from build123d import *

# Parameters (mm, degrees)
F0_W     = 127
F0_H     = 63.5
F1_DEPTH = 12.7
F2_W     = 127
F2_H     = 12.7
F3_DEPTH = 44.45
F5_DEPTH = 57.15
F6_R     = 12.7
F7_DEPTH = 44.45
F8_R     = 5.08
F9_DEPTH = 25.4


with BuildPart() as f1:
    # F0 (on Front) → F1 (new body)
    with BuildSketch(Plane.XZ):
        with Locations((63.5, 31.75)):
            Rectangle(F0_W, F0_H)
    extrude(amount=F1_DEPTH)

    # F2 (on face) → F3 (join)
    with BuildSketch(Plane.XZ.offset(12.7)):
        with Locations((63.5, 6.35)):
            Rectangle(F2_W, F2_H)
    extrude(amount=F3_DEPTH)

    # F4 (on face) → F5 (join)
    with BuildSketch(Plane.XZ.offset(57.15)):
        Polygon((31.75, -21.59), (63.5, -21.59), (95.25, -21.59), (95.25, -11.3792), (76.2, -11.3792), (76.2, 0), (63.5, 0), (50.8, 0), (50.8, -11.3792), (31.75, -11.3792), align=None)
    extrude(amount=-F5_DEPTH)

    # F6 (on face) → F7 (join)
    with BuildSketch(Plane.XZ.offset(57.15)):
        with BuildLine():
            Line((42.406574, 52.250173), (15.875, 12.7))
            Line((15.875, 12.7), (111.125, 12.7))
            Line((111.125, 12.7), (84.593426, 52.250173))
            ThreePointArc((84.593426, 52.250173), (63.5, 63.5), (42.406574, 52.250173))
        make_face()
        with Locations((63.5, 38.1)):
            Circle(F6_R, mode=Mode.SUBTRACT)
    extrude(amount=-F7_DEPTH)

    # F8 (on face) → F9 (cut)
    with BuildSketch(Plane.XY.offset(63.5)):
        with Locations((63.5, -34.925)):
            Circle(F8_R)
    extrude(amount=-F9_DEPTH, mode=Mode.SUBTRACT)


solid = f1.part
Geometry check sheet. Reference: the model listing, model coordinates, mm. A direction names the side the tool comes from. Give positions to 0.01 mm unless a question says otherwise; leave off trailing zeros. Write each loop counter-clockwise with the first axis right and the second up, starting at its lowest first coordinate (ties: lowest second). Pieces come first, ordered by that corner, then holes. Notation, with made-up numbers: (22, 37) - (51, 37) arc R21 ccw to (51, 74) - close; hole circle Ø9 at (5.5, 0). An arc over 180 degrees is marked (long way). Put each result on its own line as item: value.
1. Sectioned sample at C-C, the plane z = 16. Enter the section's corners in (x, y).
Ans:
outline: (0, -12.7) - (18.09, -12.7) - (18.09, -57.15) - (108.91, -57.15) - (108.91, -12.7) - (127, -12.7) - (127, 0) - (0, 0) - close
2. Sectioned sample at A-A, the plane y = -17. Enter the section's corners in (x, z) (3 decimals), plus the area to 3 significant figures.
Ans:
outline: (0, 0) - (50.8, 0) - (50.8, -11.379) - (31.75, -11.379) - (31.75, -21.59) - (95.25, -21.59) - (95.25, -11.379) - (76.2, -11.379) - (76.2, 0) - (127, 0) - (127, 12.7) - (111.125, 12.7) - (84.593, 52.25) arc R25.4 ccw to (42.407, 52.25) - (15.875, 12.7) - (0, 12.7) - close; hole circle Ø25.4 at (63.5, 38.1)
area: 5,100 mm²
3. Draft check along Y on faces 1 (the flat face through (63, -57.15, 12)), 2 (the cylindrical face through (68.345, -33.399, 56.717)), 3 (the flat face through (29.327, -35.236, 32.752)). Enter one of: +Y half, -Y half, draft (parallel to the pull), parting line (faces both ways), or undercut.
Ans:
face 1: -Y half
face 2: undercut
face 3: draft
4. Set-up check for faces 4 (the flat face through (25, -28, 0)), 5 (the flat face through (31.75, -29, -16)), 6 (the flat face through (109, -12.7, 44)): record each of +Z, -Z, +X, -X, +Y, -Y from which the full face is reachable in a straight line by a thin tool's end or side.
Ans:
face 4: -X, +Y, -Y
face 5: -Z, -X, +Y, -Y
face 6: +Z, +X, -Y
5. Go/stop test with flat-tipped pins: pin 1 (10 mm diameter, centred on y = -41.5, z = 47, fed in from +X); pin 2 (3 mm diameter, centred on y = -26.5, z = 37.5, fed in from +X); pin 3 (4 mm diameter, centred on y = -31, z = 16.5, fed in from +X); pin 4 (5.5 mm diameter, centred on x = 83.5, y = -15, fed in from +Z). Record where each tip stops, or that it passes through.
Ans:
pin 1: stops at x = 91.47
pin 2: stops at x = 95.49
pin 3: stops at x = 109.92
pin 4: stops at z = 63.5
6. Sectioned sample at B-B, the plane x = 87. Enter the section's corners in (y, z), plus the area to 3 significant figures.
Ans:
outline: (-57.15, -21.59) - (0, -21.59) - (0, -11.38) - (-57.15, -11.38) - close; (-57.15, 0) - (0, 0) - (0, 63.5) - (-12.7, 63.5) - (-12.7, 48.66) - (-57.15, 48.66) - close
area: 3,550 mm²
7. Sectioned sample at D-D, the plane y = -9.5. Enter the section's corners in (x, z), plus the area to 3 significant figures.
Ans:
outline: (0, 0) - (50.8, 0) - (50.8, -11.38) - (31.75, -11.38) - (31.75, -21.59) - (95.25, -21.59) - (95.25, -11.38) - (76.2, -11.38) - (76.2, 0) - (127, 0) - (127, 63.5) - (0, 63.5) - close
area: 9,000 mm²
8. Thickness scan on line 1 (Z direction, x = 63, y = -44); line 2 (Y direction, x = 63.5, z = 57.25) (3 decimals); line 3 (Y direction, x = 96, z = 48). Record the ranges inside material, lowest first.
Ans:
line 1: z = -21.59 to 25.41, 50.79 to 63.5
line 2: y = -57.15 to -40.005, -29.845 to 0
line 3: y = -12.7 to 0
